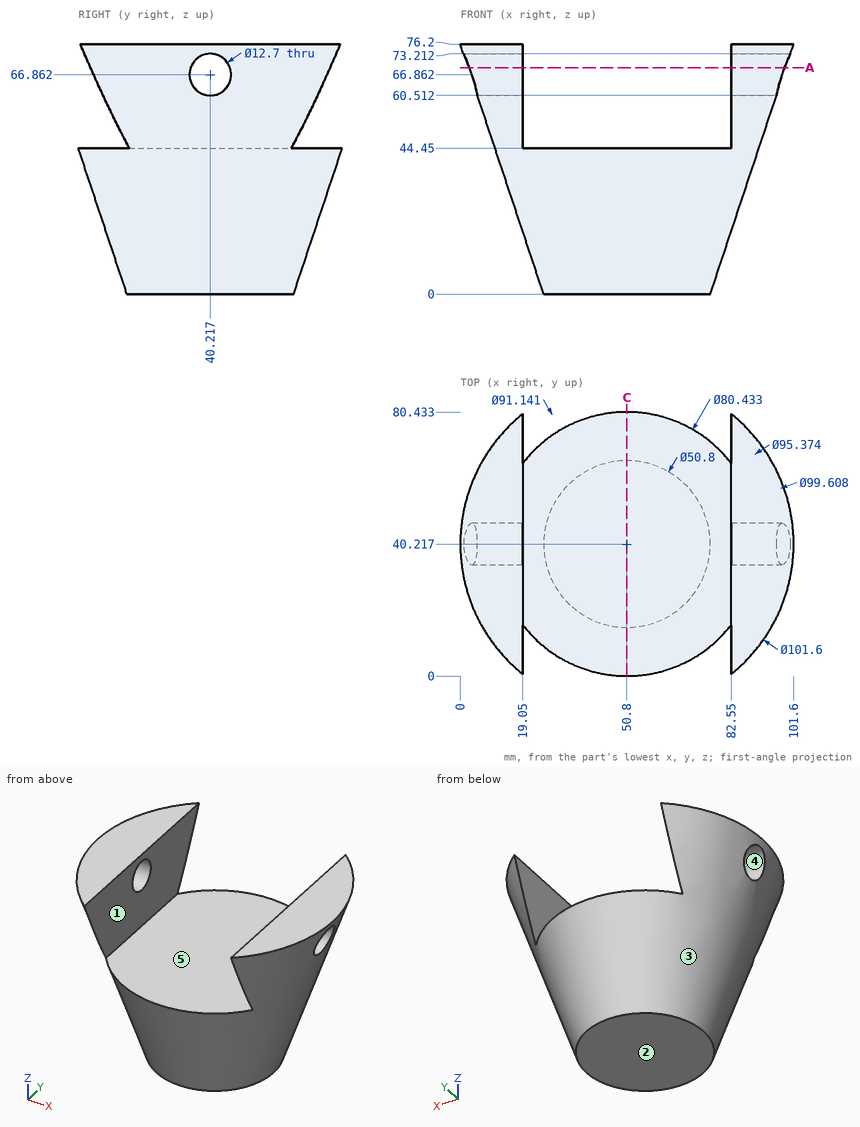
Could you check a few things on this drawing? It's one solid part, dimensions in mm from its lowest x, y, z. A direction names the side the tool comes from. Give positions to 0.01 mm unless a question says otherwise; leave off trailing zeros. Order: outer loops, then holes, each group sorted by start corner. A loop starts at its lowest first (then second) coordinate and runs counter-clockwise, first axis right, second up. Notation, with made-up numbers: (14.5, -31.5) - (36.5, -31.5) arc R27 ccw to (36.5, 0.5) - close; hole circle Ø1 at (37.25, 29.25). An arc over 180 degrees is marked (long way). Return JSON: item names as keys, results as strings. Group by question number.
Q1. Suppose I cut it at C-C, the plane x = 50.8. Please give me the cut outline in (y, z), and give its area (3 significant figures).
Q2. Thinking about a two-plate mould opening in X: for the marked faces 3, 4 and 5, which applies, pulls with the +X half, pulls with the -X half, needs draft (parallel to the pull), parting line crosses it, or undercut?
Q3. Suppose I cut it at A-A, the plane z = 69. State how many separate pieces and enclosed holes the cut face has, and give its area (3 significant figures).
Q4. Which directions (+Z, -Z, +X, -X, +Y, -Y) give clear straight access to the entire face, cutting with the end or side of a thin tool? Please do the marked faces 1 and 2.
Q5. Will these pins go through, and if not, where does the flat tip stop? pin 1 Ø16.5 at (y, z) = (40.22, 66.86) entering from +X; pin 2 Ø5 at (x, y) = (75, 32) entering from +Z; pin 3 Ø1 at (x, z) = (54, 12.5) entering from +Y (1 decimal).
Resolved:
{
 "1": {"outline": "(0, 44.45) - (14.82, 0) - (65.62, 0) - (80.43, 44.45) - close", "area": "2,920 mm2"},
 "2": {"face 3": "parting line crosses it", "face 4": "needs draft", "face 5": "undercut"},
 "3": {"separate pieces": "4", "enclosed holes": "0", "area": "1,290 mm2"},
 "4": {"face 1": "+Z, +Y, -Y", "face 2": "-Z, +X, -X, +Y, -Y"},
 "5": {"pin 1": "stops at x = 101.24", "pin 2": "stops at z = 44.45", "pin 3": "stops at y = 69.8"}
}
